Autodesk Inventor part; units mm, degrees
ref_plane "YZ Plane" through (0, 0, 0) normal (1, 0, 0) x (0, 1, 0)
ref_plane "XZ Plane" through (0, 0, 0) normal (0, 1, 0) x (-1, 0, 0)
ref_plane "XY Plane" through (0, 0, 0) normal (0, 0, 1) x (1, 0, 0)
sketch "Szkic1" plane through (0, 0, 0) normal (0, 1, 0) x (-1, 0, 0)
  circle A0 centre (0, 0) radius 4.1
  line L0 (0, 7) -> (0, -7)
  line L1 (0, -7) -> (-11, -7)
  line L2 (-11, -7) -> (-11, 7)
  line L3 (-11, 7) -> (0, 7)
  line L4 (-11, 7) -> (-6, 7)
  line L5 (-6, -7) -> (-11, -7)
  line L6 (-11, -7) -> (-11, 7)
  circle A1 centre (0, 0) radius 6
  line L7 (-6, -7) -> (-6, 7)
  point P0 (0, -6)
  point P1 (0, 6)
  point P2 (0, -4.1)
  point P3 (0, 4.1)
  point P4 (-6, 0)
  dimension "d0" = 8.2
  dimension "d1" = 14
  dimension "d2" = 11
  dimension "d3" = 7
  dimension "d6" = 0
  dimension "d7" = 5
  dimension "d8" = 12
  dimension "d15" = 5
extrude "Wyciągnięcie proste4" add sketch "Szkic1" against normal blind 20 contours A0 L0 A1 | A0 L0 A1
extrude "Wyciągnięcie proste5" add sketch "Szkic1" along normal mid plane 2 contours A0 L0 | A0 L0 A1 | L0 A0 | A0 L0 A1
extrude "Wyciągnięcie proste6" add sketch "Szkic1" along normal blind 1 contours A1 L7 L3 L0 | L0 L1 L7 A1
extrude "Wyciągnięcie proste7" add sketch "Szkic1" along normal blind 10 contours L7 L1 L2 L3
extrude "Wyciągnięcie proste8" add sketch "Szkic1" against normal blind 20 contours A1 L7 L3 L0 | L0 L1 L7 A1
extrude "Wyciągnięcie proste9" add sketch "Szkic1" against normal blind 13 contours L7 L1 L2 L3
sketch "Szkic5" plane through (0, -20, 7) normal (0, 0, 1) x (1, 0, 0)
  line L0 (6, 21) -> (0, 21)
  line L1 (6, 21) -> (6, 30)
  line L2 (0, 21) -> (6, 30)
  line L3 (6, 30) -> (11, 37.5)
  line L4 (11, 7) -> (11, 30)
  line L5 (11, 30) -> (11, 37.5)
  line L6 (11, 30) -> (6, 30)
  line L7 (6, 30) -> (6, 21)
  line L8 (6, 30) -> (6, 21)
  line L9 (0, 21) -> (6, 21)
  point P0 (0, 20)
extrude "Wyciągnięcie proste10" add sketch "Szkic5" against normal blind 14
properties part number "chwytak_rurki"
The listing builds one solid part. Answer for the finished solid, in the listing's coordinates (mm). A direction names the side the tool comes from. Give positions to 0.01 mm unless a question says otherwise; leave off trailing zeros. Loops run counter-clockwise (first coordinate to the right, second up) from the corner with the lowest first, then second, coordinate; pieces in that order, holes last. Notation, with made-up numbers: (-29.5, -6.75) - (-12.5, -6.75) arc R33 cw to (-12.5, 21.25) - close; hole circle Ø3 at (87, 7.25). An arc over 180 degrees is marked (long way). Answer as CSV lines item,"result". Start each with the question number.
Item 1: A cutting plane is placed at C-C on x = 9.25. Determine the outline of the cut face in (y, z) (3 decimals), then the cut area to 3 significant figures.
Item 2: For faces 4 (the face through (0, -1, 0)), 5 (the face through (-2, 1, 0)), 6 (the face through (6, -16, 0)), 7 (the face through (0, -9.6, -6.5)), 8 (the face through (0, -9.6, 6.5)), determine the directions among +Z, -Z, +X, -X, +Y, -Y from which every point of the face is accessible in a straight line to the end or side of a thin tool.
Item 3: The mould has two halves that part along X. Classify faces 1 (the face through (-6, -9, 0)), 2 (the face through (5, -5, -7)), 3 (the face through (0.534, -10.367, 4.065)): +X half, -X half, draft (parallel to the pull), parting line (faces both ways), or undercut.
Item 4: A cutting plane is placed at D-D on z = -3. Determine the outline of the cut face in (x, y).
Item 5: A cutting plane is placed at A-A on y = -6. Determine the outline of the cut face in (x, z), then the cut area to 3 significant figures.
Item 6: A cutting plane is placed at B-B on z = 0. Determine the outline of the cut face in (x, y), then the cut area to 3 significant figures.
Item 7: Find the intervals of material crossed by line 1 (X direction, y = -9.75, z = 0); line 2 (Y direction, x = -2.75, z = -1.75); line 3 (X direction, y = -7.5, z = 3.5), in increasing order. Write a range as from..to.
Item 8: Each of these flat-tipped pins is pushed along its axis until it touches: pin 1 (0.8 mm diameter, centred on y = -10, z = 6.5, fed in from -X); pin 2 (2 mm diameter, centred on y = -17, z = 1, fed in from +X); pin 3 (2 mm diameter, centred on x = 4, z = 4, fed in from +Y). Where does it stop, or does it pass through?
Found:
1,outline,"(-13, -7) - (14.875, -7) - (14.875, 7) - (-13, 7) - close"
1,area,"390 mm^2"
2,face 4,"-Y"
2,face 5,"+Z, -Z, -X, +Y"
2,face 6,"+Z, -Z, +X, -Y"
2,face 7,"-Z, -X, +Y, -Y"
2,face 8,"+Z, -X, +Y, -Y"
3,face 1,"-X half"
3,face 2,"draft"
3,face 3,"undercut"
4,outline,"(-5.2, -20) - (-2.79, -20) - (-2.79, -1) - (2.79, -1) - (2.79, -20) - (6, -20) - (6, -13) - (11, -13) - (11, 17.5) - (0, 1) - (-5.2, 1) - close"
5,outline,"(0, -7) - (11, -7) - (11, 7) - (0, 7) - (0, 6) arc R6 ccw to (0, -6) - close; hole circle Ø8.2 at (0, 0)"
5,area,"158 mm^2"
6,outline,"(-6, -20) - (-4.1, -20) - (-4.1, -1) - (4.1, -1) - (4.1, -20) - (6, -20) - (6, -13) - (11, -13) - (11, 17.5) - (0, 1) - (-6, 1) - close"
6,area,"257 mm^2"
7,line 1,"x = -6..-4.1, 4.1..11"
7,line 2,"y = -1..1"
7,line 3,"x = -4.87..-2.14, 2.14..11"
8,pin 1,"stops at x = 0"
8,pin 2,"stops at x = 6"
8,pin 3,"stops at y = 8.5"
